The model under review builds one solid part; all positions refer to its coordinate system, in mm. Face numbers are marked on the shaded views. A direction names the side the tool comes from. Give positions to 0.01 mm unless a question says otherwise; leave off trailing zeros. Loops run counter-clockwise (first coordinate to the right, second up) from the corner with the lowest first, then second, coordinate; pieces in that order, holes last. Notation, with made-up numbers: (34, -25.5) - (73, -25.5) arc R4 ccw to (73, -18.5) - close; hole circle Ø4 at (25.25, -12.5). An arc over 180 degrees is marked (long way). Return JSON: item names as keys, results as strings. Group by question number.
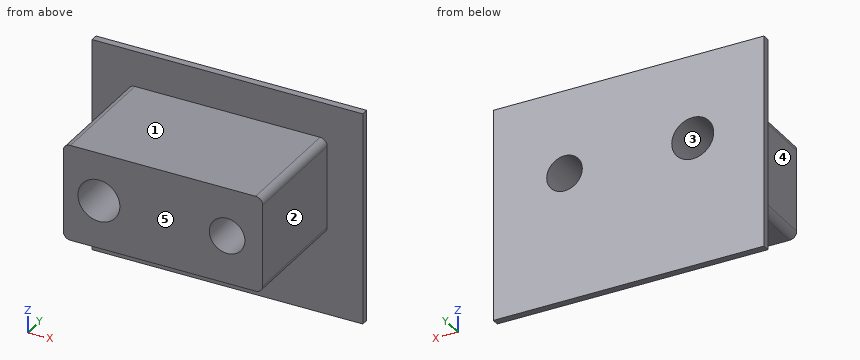
from build123d import *

# Parameters (mm, degrees)
SKETCH1_W           = 14
SKETCH1_H           = 8.2625
EXTRUDE1_DEPTH      = 3.375
SKETCH4_W           = 19
SKETCH4_H           = 11.75
EXTRUDE2_DEPTH      = 0.5
SKETCH2_W           = 1.4732
SKETCH2_H           = 16.500973173
SKETCH3_W           = 1.25
SKETCH3_H           = 20
FILLET1_R           = 0.5
SKETCH6_W           = 19
SKETCH6_H           = 0.5
BOSS_EXTRUDE2_DEPTH = 3.2


with BuildPart() as part:
    # Sketch1 → Extrude1 (new body, symmetric)
    with BuildSketch(Plane.XY):
        with Locations((0, 189.13125)):
            Rectangle(SKETCH1_W, SKETCH1_H)
    extrude(amount=EXTRUDE1_DEPTH, both=True)

    # Sketch4 → Extrude2 (add)
    with BuildSketch(Plane(origin=(0, 193.2625, 0), x_dir=(1, 0, 0), z_dir=(0, 1, 0))):
        Rectangle(SKETCH4_W, SKETCH4_H)
    extrude(amount=EXTRUDE2_DEPTH)

    # Sketch2 → Cut-Revolve1 (revolve, cut)
    with BuildSketch(Plane(origin=(9.451328919, 219.930638069, 0), x_dir=(1, 0, 0), z_dir=(0, 0, -1)), mode=Mode.PRIVATE) as cut_revolve1_sk:
        with Locations((-13.214728919, 29.739409073)):
            Rectangle(SKETCH2_W, SKETCH2_H)
    revolve(cut_revolve1_sk.sketch.rotate(Axis((-4.5, 202.803113019, 0), (0, -1, 0)), 90), axis=Axis((-4.5, 202.803113019, 0), (0, -1, 0)), mode=Mode.SUBTRACT)  # turned: the seam where the file's is

    # Sketch3 → Cut-Revolve2 (revolve, cut)
    with BuildSketch(Plane.XY, mode=Mode.PRIVATE) as cut_revolve2_sk:
        with Locations((5.125, 191.895853695)):
            Rectangle(SKETCH3_W, SKETCH3_H)
    revolve(cut_revolve2_sk.sketch.rotate(Axis((4.5, 219.496854939, 0), (0, -1, 0)), 90), axis=Axis((4.5, 219.496854939, 0), (0, -1, 0)), mode=Mode.SUBTRACT)  # turned: the seam where the file's is

    # Fillet1
    fillet1_edges = [part.edges().sort_by_distance(p)[0] for p in [
        (7, 189.13125, 3.375),
        (-7, 189.13125, 3.375),
        (7, 189.13125, -3.375),
        (-7, 189.13125, -3.375),
    ]]
    fillet(fillet1_edges, radius=FILLET1_R)

    # Sketch6 → Boss-Extrude2 (add)
    with BuildSketch(Plane(origin=(0, 0, -5.875), x_dir=(-1, 0, 0), z_dir=(0, 0, -1))):
        with Locations((0, 193.5125)):
            Rectangle(SKETCH6_W, SKETCH6_H)
    extrude(amount=BOSS_EXTRUDE2_DEPTH)


solid = part.part
Item 1: Take a section at B-B (y = 188.25). State the section outline as (x, z) points (3 decimals), then the cut area to 3 significant figures.
Item 2: Take a section at C-C (z = 0). State the section outline as (x, y) points.
Item 3: Mouldability with a two-part tool opening along Z and no side actions: class the marked faces 1, 2 and 3 as +Z half, -Z half, draft (parallel to the pull), parting line (faces both ways), or undercut.
Item 4: For L1, parallel to X at y = 191.5, z = 0; L2, parallel to Z at x = -4.5, y = 191.5 (3 decimals); L3, parallel to Y at x = -0.5, z = 5.25, list the stretches that pass through material, from the lowest coordinate up. Write a range as from..to.
Item 5: Tool access review of the marked faces 4 and 5: name each direction out of +Z, -Z, +X, -X, +Y, -Y from which nothing blocks a thin tool from reaching the whole face with its end or side.
Item 6: For P1, Ø2, axis at x = 4.5, z = 0, coming from the -Y side; P2, Ø3, axis at y = 188, z = -0.5, coming from the +X side; P3, Ø4, axis at x = 4.5, y = 191, coming from the +Z side (3 decimals); P4, Ø4, axis at x = 1, z = -6.5, coming from the -Y side, all flat-tipped, find the tip position at first contact; note any pin that passes through.
Item 7: Take a section at D-D (x = -2.75). State the section outline as (y, z) points (1 decimal).
Check sheet entries:
{
 "1": {"outline": "(-7, -2.875) arc R0.5 ccw to (-6.5, -3.375) - (6.5, -3.375) arc R0.5 ccw to (7, -2.875) - (7, 2.875) arc R0.5 ccw to (6.5, 3.375) - (-6.5, 3.375) arc R0.5 ccw to (-7, 2.875) - close; hole circle Ø2.946 at (-4.5, 0); hole circle Ø2.5 at (4.5, 0)", "area": "82.6 mm^2"},
 "2": {"outline": "(-9.5, 193.26) - (-7, 193.26) - (-7, 185) - (-5.97, 185) - (-5.97, 193.76) - (-9.5, 193.76) - close; (-3.03, 185) - (3.25, 185) - (3.25, 193.76) - (-3.03, 193.76) - close; (5.75, 185) - (7, 185) - (7, 193.26) - (9.5, 193.26) - (9.5, 193.76) - (5.75, 193.76) - close"},
 "3": {"face 1": "+Z half", "face 2": "draft", "face 3": "undercut"},
 "4": {"L1": "x = -7..-5.97, -3.03..3.25, 5.75..7", "L2": "z = -3.375..-1.473, 1.473..3.375", "L3": "y = 193.26..193.76"},
 "5": {"face 4": "+Z, -Z, -X, -Y", "face 5": "+Z, -Z, +X, -X, -Y"},
 "6": {"P1": "passes through", "P2": "stops at x = 7", "P3": "stops at z = 3.375", "P4": "stops at y = 193.26"},
 "7": {"outline": "(185, -3.4) - (193.3, -3.4) - (193.3, -9.1) - (193.8, -9.1) - (193.8, 5.9) - (193.3, 5.9) - (193.3, 3.4) - (185, 3.4) - close"}
}
